Source: CAD feature listing. Evaluate the final solid. Frame: model axes, mm. A direction names the side the tool comes from. Round coordinates to 2 decimals unless told otherwise and drop trailing zeros. Write each loop counter-clockwise with the first axis right and the second up, starting at its lowest first coordinate (ties: lowest second). Pieces come first, ordered by that corner, then holes. Notation, with made-up numbers: M 74,72 L 95,72 A19 ccw 95,100 Z; hole C -14,67 d6. An arc over 180 degrees is marked long. Answer in a Markdown table with one row per item. Add a question column.
Item 1: Contact query for flat-ended pins moving along their axis: pin 1 (5 mm diameter, centred on x = -2.18, z = -0.71, fed in from +Y); pin 2 (3 mm diameter, centred on x = -3.5, y = 2, fed in from +Z); pin 3 (4 mm diameter, centred on x = 12, y = 3.5, fed in from +Z); pin 4 (6.5 mm diameter, centred on x = 12, y = 9.5, fed in from -Z). Output: stop coordinate, or through.
Item 2: Cut plane C-C on y = 10.5. Return loops of the section in (x, z), and give its area (3 significant figures).
Item 3: Material intervals for probe 1 along Z at (x, y) = (-2, 1.5); probe 2 along Z at (x, y) = (12, 8.25); probe 3 along X at (y, z) = (6.5, -1.5), sorted ascending.
Item 4: Cut plane D-D on x = 9. Return loops of the section in (y, z) (3 decimals), and give its area (3 significant figures).
Item 5: Mould query, pull axis X, two halves, no side actions, for faces 1 (the face through (1.82, 9, 11)), 2 (the face through (-4, 0, -3)), 3 (the face through (18.8, 9.1, 39)). Classes: released by +X, released by -X, zero draft, split by the parting line, or undercut.
Item 6: Set-up query: faces 4 (the face through (-6.18, 9, 20)), 5 (the face through (11, 9, 35.287)), 6 (the face through (0.26, -2.07, -1.25)), 7 (the face through (-2, 3, 3.287)), 8 (the face through (-2, 0, -1)). Return all of +Z, -Z, +X, -X, +Y, -Y with unobstructed straight access to the full face (end or side cutting, diameter ignored); none if empty.
Item 7: Cut plane A-A on z = 40. Return loops of the section in (x, y) (3 decimals).
Item 8: Cut plane B-B on x = 15.75. Return loops of the section in (y, z) (3 decimals), and give its area (3 significant figures).
from build123d import *

# Parameters (mm, degrees)
SKETCH1_W      = 27
SKETCH1_H      = 48
EXTRUDE1_DEPTH = 12
SKETCH2_R      = 1.5
SKETCH2_R_2    = 2
SKETCH2_W      = 19
SKETCH2_H      = 40
EXTRUDE2_DEPTH = 50.510339849
SKETCH3_W      = 40
SKETCH3_H      = 6.175
EXTRUDE3_DEPTH = 53.409819068
SKETCH7_R      = 2.5
EXTRUDE7_DEPTH = 4.2


with BuildPart() as part:
    # Sketch1 → Extrude1 (new body)
    with BuildSketch(Plane(origin=(0, 0, 0), x_dir=(1, 0, 0), z_dir=(0, 1, 0))):
        with Locations((7.320293399, -19.287286064)):
            Rectangle(SKETCH1_W, SKETCH1_H)
    extrude(amount=EXTRUDE1_DEPTH)

    # Sketch2 → Extrude2 (cut, through all)
    with BuildSketch(Plane(origin=(0, 12, 0), x_dir=(1, 0, 0), z_dir=(0, 1, 0))):
        with Locations(Location((-2.179706601, 0.712713936, 0), (0, 0, 270))):
            Circle(SKETCH2_R)
        with Locations(Location((16.820293399, -39.287286064, 0), (0, 0, 270))):
            Circle(SKETCH2_R_2)
        with Locations((11.320293399, -15.287286064)):
            Rectangle(SKETCH2_W, SKETCH2_H)
    extrude(amount=-EXTRUDE2_DEPTH, mode=Mode.SUBTRACT)

    # Sketch3 → Extrude3 (cut, through all)
    with BuildSketch(Plane(origin=(20.820293399, 0, 0), x_dir=(0, 0, -1), z_dir=(1, 0, 0))):
        with Locations((-23.287286064, 3.0875)):
            Rectangle(SKETCH3_W, SKETCH3_H)
    extrude(amount=-EXTRUDE3_DEPTH, mode=Mode.SUBTRACT)

    # Sketch7 → Extrude7 (add)
    with BuildSketch(Plane.XZ):
        with Locations(Location((-2.179706601, -0.712713936, 0), (0, 0, 90))):
            Circle(SKETCH7_R)
    extrude(amount=EXTRUDE7_DEPTH)


solid = part.part
Results below:
| question | item | result |
|---|---|---|
| 1 | pin 1 | y = 12 |
| 1 | pin 2 | z = 3.29 |
| 1 | pin 3 | through |
| 1 | pin 4 | z = 35.29 |
| 2 | outline | M -6.18,-4.71 L 1.82,-4.71 L 1.82,35.29 L 20.82,35.29 L 20.82,43.29 L -6.18,43.29 Z; hole C -2.18,-0.71 d3; hole C 16.82,39.29 d4 |
| 2 | area | 516 mm2 |
| 3 | probe 1 | -4.71 to -2.2, 0.78 to 3.29 |
| 3 | probe 2 | 35.29 to 43.29 |
| 3 | probe 3 | -6.18 to -3.46, -0.9 to 1.82 |
| 4 | outline | M 6.175,35.287 L 12,35.287 L 12,43.287 L 6.175,43.287 Z |
| 4 | area | 46.6 mm2 |
| 5 | face 1 | released by +X |
| 5 | face 2 | zero draft |
| 5 | face 3 | undercut |
| 6 | face 4 | +Z, -Z, -X, +Y, -Y |
| 6 | face 5 | -Z, +X, +Y, -Y |
| 6 | face 6 | -Y |
| 6 | face 7 | +Z, +X, -X, -Y |
| 6 | face 8 | +Y |
| 7 | outline | M -6.18,6.175 L 14.952,6.175 L 14.952,12 L -6.18,12 Z; M 18.689,6.175 L 20.82,6.175 L 20.82,12 L 18.689,12 Z |
| 8 | outline | M 6.175,35.287 L 12,35.287 L 12,37.598 L 6.175,37.598 Z; M 6.175,40.977 L 12,40.977 L 12,43.287 L 6.175,43.287 Z |
| 8 | area | 26.9 mm2 |
